Work out the finished part from the listing and answer in its coordinate system (mm). A direction names the side the tool comes from. Give positions to 0.01 mm unless a question says otherwise; leave off trailing zeros. Loops run counter-clockwise (first coordinate to the right, second up) from the corner with the lowest first, then second, coordinate; pieces in that order, holes last.
from build123d import *

# Parameters (mm, degrees)
ESBO_O1_W                  = 50
ESBO_O1_H                  = 80
RESSALTO_EXTRUS_O1_DEPTH   = 70
CORTE_EXTRUS_O1_DEPTH      = 118.473401245
CORTE_EXTRUS_O1_DEPTH_BACK = 118.473401245
ESBO_O2_W                  = 40
ESBO_O2_H                  = 40
CHANFRO1_SIZE              = 15
FILETE1_R                  = 10


with BuildPart() as part:
    # Esboço1 → Ressalto-extrusão1 (new body)
    with BuildSketch(Plane(origin=(0, 0, 0), x_dir=(1, 0, 0), z_dir=(0, 1, 0))):
        with Locations((25, 40)):
            Rectangle(ESBO_O1_W, ESBO_O1_H)
    extrude(amount=RESSALTO_EXTRUS_O1_DEPTH)

    # Esboço2 → Corte-extrusão1 (cut, two sides: drawn at the far end of the back side and taken through both)
    with BuildSketch(Plane(origin=(50, 0, 0), x_dir=(0, 0, -1), z_dir=(1, 0, 0)).offset(-CORTE_EXTRUS_O1_DEPTH_BACK)):
        with Locations((20, 50)):
            Rectangle(ESBO_O2_W, ESBO_O2_H)
    extrude(amount=CORTE_EXTRUS_O1_DEPTH + CORTE_EXTRUS_O1_DEPTH_BACK, mode=Mode.SUBTRACT)

    # Chanfro1
    chanfro1_edges = [part.edges().sort_by_distance(p)[0] for p in [
        (25, 70, -40),
    ]]
    chamfer(chanfro1_edges, length=CHANFRO1_SIZE)

    # Filete1
    filete1_edges = [part.edges().sort_by_distance(p)[0] for p in [
        (25, 70, -80),
        (25, 30, 0),
    ]]
    fillet(filete1_edges, radius=FILETE1_R)


solid = part.part
Item 1: Consider line 1 (Y direction, x = 48, z = -10.5); line 2 (Z direction, x = 48.5, y = 20.5); line 3 (Z direction, x = 32, y = 33). Determine where each line is inside the solid, lowest interval first.
Item 2: Flat-ended cylindrical pins translate along their axes: pin 1 Ø12 at (y, z) = (49.5, -37) entering from +X; pin 2 Ø5 at (x, y) = (20, 26) entering from +Z; pin 3 Ø1.5 at (x, y) = (24, 37) entering from +Z; pin 4 Ø1 at (x, z) = (43.5, -17) entering from +Y. Find the tip coordinate at first contact, or state that the pin passes through.
Item 3: Find section A-A, the plane x = 43. Write down the section's boundary in (y, z).
Item 4: Find section B-B, the plane z = -18.5. Write down the section's boundary in (x, y), plus the area to 3 significant figures.
Item 5: Find section C-C, the plane y = 43. Write down the section's boundary in (x, z), plus the area to 3 significant figures.
Item 6: For faces 1 (the face through (25, 0, -41)), 2 (the face through (25, 42, -40)), determine the directions among +Z, -Z, +X, -X, +Y, -Y from which every point of the face is accessible in a straight line to the end or side of a thin tool.
Ans:
1. line 1: y = 0 to 30
1. line 2: z = -80 to -0.01
1. line 3: z = -80 to -40
2. pin 1: stops at x = 50
2. pin 2: stops at z = -0.63
2. pin 3: stops at z = -40
2. pin 4: stops at y = 30
3. outline: (0, -80) - (60, -80) arc R10 ccw to (70, -70) - (70, -55) - (55, -40) - (30, -40) - (30, -10) arc R10 ccw to (20, 0) - (0, 0) - close
4. outline: (0, 0) - (50, 0) - (50, 30) - (0, 30) - close
4. area: 1,500 mm2
5. outline: (0, -80) - (50, -80) - (50, -40) - (0, -40) - close
5. area: 2,000 mm2
6. face 1: +Z, -Z, +X, -X, -Y
6. face 2: +Z, +X, -X, +Y
